Design review of the part built by this model. Coordinates are the model's own, in mm. A direction names the side the tool comes from. Round coordinates to 2 decimals unless told otherwise and drop trailing zeros. Loops run counter-clockwise (first coordinate to the right, second up) from the corner with the lowest first, then second, coordinate; pieces in that order, holes last. Notation, with made-up numbers: (18, -26) - (77, -26) arc R16 cw to (77, 2) - close; hole circle Ø9 at (66, 2). An arc over 180 degrees is marked (long way). Return JSON: item names as keys, results as strings. Group by question number.
(1) We need section D-D, the plane z = 0.75. Write out the cut boundary in (x, y) (3 decimals).
(2) Wall thickness on L1, parallel to Y at x = -3.05, z = 0.55; L2, parallel to Z at x = 4, y = 9; L3, parallel to Z at x = -3.25, y = 1.75: over which ranges is each line inside the solid? List them lowest first. Write a range as [from, to].
(3) The part is to be moulded in two halves that separate along Y. For faces 4 (the cylindrical face through (-2.55, 3.28, 3.11)), 5 (the cylindrical face through (-8.47, 8.25, 4.41)), 6 (the cylindrical face through (-13.074, 1.12, 0.887)), say which applies: pulls with the +Y half, pulls with the -Y half, needs draft (parallel to the pull), parting line crosses it, or undercut.
(4) We need section C-C, the plane z = 2.5. Write out the cut boundary in (x, y), and give its area (3 significant figures).
(5) We need section B-B, the plane y = 3.25. Write out the cut boundary in (x, z) (3 decimals).
(6) We need section A-A, the plane x = -3.05. Write out the cut boundary in (y, z), and give its area (3 significant figures).
(7) Clearance check with flat-ended pins moving along their axes: pin 1 (1.5 mm diameter, centred on x = -11, z = 2, fed in from +Y); pin 2 (2 mm diameter, centred on y = 5.5, z = 4.5, fed in from +X); pin 3 (8 mm diameter, centred on x = -1.5, y = 5, fed in from +Z). State where each tip first meets the part, or that it passes through.
(8) For faces 1 (the cylindrical face through (-3.55, 3.22, 3.11)), 2 (the flat face through (-3, 1.25, 3)), 3 (the cylindrical face through (-6.33, 9.65, 4.41)), list the 3-axis set-ups (+Z, -Z, +X, -X, +Y, -Y) from which the entire face can be reached by the end or side of a thin tool; tool diameter is ignored.
from build123d import *

# Parameters (mm, degrees)
SKETCH_1_R      = 0.925
EXTRUDE_1_DEPTH = 1.8
SKETCH_2_R      = 0.925
EXTRUDE_2_DEPTH = 1.8
EXTRUDE_3_DEPTH = 5.3
EXTRUDE_4_DEPTH = 2.65


with BuildPart() as part:
    # Sketch 1 → Extrude 1 (new body)
    with BuildSketch(Plane.XY):
        with BuildLine():
            Line((-8.55, 8.25), (2.45, 8.25))
            ThreePointArc((2.45, 8.25), (7.45, 3.25), (2.45, -1.75))
            Line((2.45, -1.75), (-8.55, -1.75))
            ThreePointArc((-8.55, -1.75), (-13.55, 3.25), (-8.55, 8.25))
        make_face()
        with Locations((-8.55, 3.25)):
            Circle(SKETCH_1_R, mode=Mode.SUBTRACT)
        with Locations((2.45, 3.25)):
            Circle(SKETCH_1_R, mode=Mode.SUBTRACT)
    extrude(amount=EXTRUDE_1_DEPTH)

    # Sketch 2 → Extrude 2 (add)
    with BuildSketch(Plane.XY.offset(1.8)):
        with BuildLine():
            Line((-12.299646462, 6.55758997), (-6.57492094, 13.047420027))
            ThreePointArc((-6.57492094, 13.047420027), (-3.05, 14.638399767), (0.47492094, 13.047420027))
            Line((0.47492094, 13.047420027), (6.199646462, 6.55758997))
            ThreePointArc((6.199646462, 6.55758997), (4.506945569, 7.807299082), (2.45, 8.25))
            Line((2.45, 8.25), (-8.55, 8.25))
            ThreePointArc((-8.55, 8.25), (-10.606945569, 7.807299082), (-12.299646462, 6.55758997))
        make_face()
        with Locations((-3.05, 10.863062049)):
            Circle(SKETCH_2_R, mode=Mode.SUBTRACT)
    extrude(amount=-EXTRUDE_2_DEPTH)

    # Sketch 3 → Extrude 3 (add)
    with BuildSketch(Plane.XY.offset(1.8)):
        with BuildLine():
            Line((-7.116209234, 12.433789028), (-11.416941699, 7.558267449))
            Line((-11.416941699, 7.558267449), (-11.319997249, 7.412585163))
            ThreePointArc((-11.319997249, 7.412585163), (-8.425967454, 8.248461356), (-5.576956996, 7.270076529))
            Line((-5.576956996, 7.270076529), (-5.044384077, 7.990208692))
            ThreePointArc((-5.044384077, 7.990208692), (-6.342261306, 9.683286753), (-6.415115625, 11.815349339))
            Line((-6.415115625, 11.815349339), (-7.116209234, 12.433789028))
        make_face()
    extrude(amount=EXTRUDE_3_DEPTH)

    # Sketch 3_3 → Extrude 4 (add)
    with BuildSketch(Plane.XY.offset(1.8)):
        with BuildLine():
            ThreePointArc((-2.132575695, 5.25), (-2.55, 3.25), (-2.132575695, 1.25))
            Line((-2.132575695, 1.25), (-3.967424305, 1.25))
            ThreePointArc((-3.967424305, 1.25), (-3.55, 3.25), (-3.967424305, 5.25))
            Line((-3.967424305, 5.25), (-2.132575695, 5.25))
        make_face()
    extrude(amount=EXTRUDE_4_DEPTH)


solid = part.part
Solutions:
{
 "1": {"outline": "(-12.3, 6.558) arc R5 ccw to (-8.55, -1.75) - (2.45, -1.75) arc R5 ccw to (6.2, 6.558) - (0.475, 13.047) arc R4.7 ccw to (-6.575, 13.047) - close; hole circle Ø1.85 at (-8.55, 3.25); hole circle Ø1.85 at (-3.05, 10.863); hole circle Ø1.85 at (2.45, 3.25)"},
 "2": {"L1": "[-1.75, 9.94], [11.79, 14.64]", "L2": "[0, 1.8]", "L3": "[0, 4.45]"},
 "3": {"face 4": "undercut", "face 5": "pulls with the -Y half", "face 6": "parting line crosses it"},
 "4": {"outline": "(-11.42, 7.56) - (-11.32, 7.41) arc R5 cw to (-5.58, 7.27) - (-5.04, 7.99) arc R3.5 cw to (-6.42, 11.82) - (-7.12, 12.43) - close; (-3.97, 1.25) - (-2.13, 1.25) arc R5 cw to (-2.13, 5.25) - (-3.97, 5.25) arc R5 cw to start", "area": "17.9 mm^2"},
 "5": {"outline": "(-13.55, 0) - (-9.475, 0) - (-9.475, 1.8) - (-13.55, 1.8) - close; (-7.625, 0) - (1.525, 0) - (1.525, 1.8) - (-2.55, 1.8) - (-2.55, 4.45) - (-3.55, 4.45) - (-3.55, 1.8) - (-7.625, 1.8) - close; (3.375, 0) - (7.45, 0) - (7.45, 1.8) - (3.375, 1.8) - close"},
 "6": {"outline": "(-1.75, 0) - (9.94, 0) - (9.94, 1.8) - (5.25, 1.8) - (5.25, 4.45) - (1.25, 4.45) - (1.25, 1.8) - (-1.75, 1.8) - close; (11.79, 0) - (14.64, 0) - (14.64, 1.8) - (11.79, 1.8) - close", "area": "36.8 mm^2"},
 "7": {"pin 1": "y = 8.88", "pin 2": "x = -2.13", "pin 3": "z = 4.45"},
 "8": {"face 1": "+Z, -X", "face 2": "+Z, +X, -X, -Y", "face 3": "+Z, +X"}
}
